Can you work these out from the model? Positions are in its coordinate system, mm. Round coordinates to 2 decimals unless told otherwise and drop trailing zeros. Loops run counter-clockwise (first coordinate to the right, second up) from the corner with the lowest first, then second, coordinate; pieces in that order, holes last.
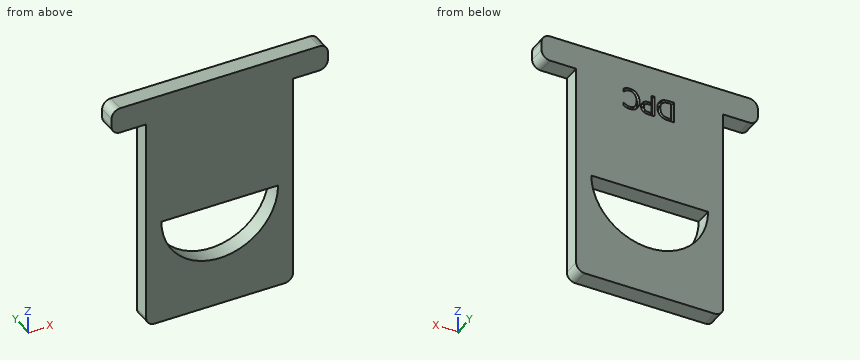
Autodesk Inventor part; units mm, degrees
ref_plane "YZ Plane" through (0, 0, 0) normal (1, 0, 0) x (0, 1, 0)
ref_plane "XZ Plane" through (0, 0, 0) normal (0, 1, 0) x (-1, 0, 0)
ref_plane "XY Plane" through (0, 0, 0) normal (0, 0, 1) x (1, 0, 0)
sketch "Sketch1" plane through (0, 0, 0) normal (0, 1, 0) x (-1, 0, 0)
  line L0 (-17, 25) -> (17, 25)
  line L1 (17, 25) -> (17, -25)
  line L2 (17, -25) -> (-17, -25)
  line L3 (-17, -25) -> (-17, 25)
  line L4 (-17, 25) -> (17, -25) construction
  line L5 (17, 25) -> (-17, -25) construction
  line L6 (9, -17) -> (9, 17)
  line L7 (9, 17) -> (-9, 17)
  line L8 (-9, 17) -> (-9, -17)
  line L9 (-9, -17) -> (9, -17)
  line L10 (-25, 31) -> (25, 31)
  line L11 (25, 31) -> (25, 25)
  line L12 (25, 25) -> (-25, 25)
  line L13 (-25, 25) -> (-25, 31)
  line L14 (-25, 31) -> (25, 25) construction
  line L15 (25, 31) -> (-25, 25) construction
  point P0 (0, 0)
  point P1 (0, 28)
  point P2 (0, 25)
  dimension "d0" = 34
  dimension "d1" = 50
  dimension "d2" = 8
  dimension "d3" = 50
  dimension "d4" = 6
extrude "Extrusion1" add sketch "Sketch1" along normal blind 4 contours L12 L13 L10 L11 L0 | L0 L1 L2 L3 | L9 L8 L7 L6
sketch "Sketch2" plane through (0, 4, 0) normal (0, 1, 0) x (1, 0, 0)
  line L0 (25, -25) -> (17, -25)
  line L1 (17, -25) -> (17, 25)
  line L2 (17, 25) -> (-17, 25)
  line L3 (-17, 25) -> (-17, -25)
  line L4 (-17, -25) -> (-25, -25)
  line L5 (-25, -25) -> (-25, -31)
  line L6 (-25, -31) -> (25, -31)
  line L7 (25, -31) -> (25, -25)
  line L8 (13.5, 17) -> (-13.5, 17)
  line L9 (-13.5, 17) -> (-13.5, -17)
  line L10 (-13.5, -17) -> (13.5, -17)
  line L11 (13.5, -17) -> (13.5, 17)
  line L12 (13.5, 17) -> (-13.5, -17) construction
  line L13 (-13.5, 17) -> (13.5, -17) construction
  circle A0 centre (0, 0.2783) radius 13.5
  line L14 (-13.5, 0.2783) -> (13.5, 0.2783)
  point P0 (-1.4697, 0.3)
  point P1 (1.4697, 0.3)
  point P2 (13.5, 0)
  point P3 (-13.5, 0)
  dimension "d7" = 27
  dimension "d8" = 34
extrude "Extrusion2" cut sketch "Sketch2" against normal through all contours L14 A0 picked at (2.5563, 3.9817)
sketch "Sketch3" plane through (0, 4, 0) normal (0, 1, 0) x (1, 0, 0)
  line L0 (-6.091, -19.1641) -> (19.1348, -19.1641) construction
  line L1 (19.1348, -19.1641) -> (19.1348, -24.3512) construction
  line L2 (19.1348, -24.3512) -> (-6.091, -24.3512) construction
  line L3 (-6.091, -24.3512) -> (-6.091, -19.1641) construction
  spline S0 degree 2 poles (-1.7599, -21.6886) (-1.7599, -22.3553) (-2.3003, -23.4282) (-2.7539, -23.728) knots 0 0 0 1 2 2 2
  spline S1 degree 2 poles (-2.7539, -23.728) (-3.1247, -23.9607) (-3.886, -24.1185) (-4.4777, -24.1185) knots 0 0 0 1 2 2 2
  line L4 (-4.4777, -24.1185) -> (-5.598, -24.1185)
  line L5 (-5.598, -24.1185) -> (-5.598, -19.2508)
  line L6 (-5.598, -19.2508) -> (-4.4895, -19.2508)
  spline S2 degree 2 poles (-4.4895, -19.2508) (-3.8032, -19.2508) (-3.0221, -19.456) (-2.746, -19.6374) knots 0 0 0 1 2 2 2
  spline S3 degree 2 poles (-2.746, -19.6374) (-2.2766, -19.949) (-1.7599, -20.9786) (-1.7599, -21.6886) knots 0 0 0 1 2 2 2
  spline S4 degree 2 poles (-2.4344, -21.6807) (-2.4344, -21.1206) (-2.8052, -20.3277) (-3.172, -20.1029) knots 0 0 0 1 2 2 2
  spline S5 degree 2 poles (-3.172, -20.1029) (-3.4324, -19.949) (-4.0201, -19.811) (-4.458, -19.811) knots 0 0 0 1 2 2 2
  line L7 (-4.458, -19.811) -> (-4.9511, -19.811)
  line L8 (-4.9511, -19.811) -> (-4.9511, -23.5584)
  line L9 (-4.9511, -23.5584) -> (-4.458, -23.5584)
  spline S6 degree 2 poles (-4.458, -23.5584) (-4.028, -23.5584) (-3.3772, -23.4203) (-3.1129, -23.2349) knots 0 0 0 1 2 2 2
  spline S7 degree 2 poles (-3.1129, -23.2349) (-2.7736, -23.0061) (-2.4344, -22.2488) (-2.4344, -21.6807) knots 0 0 0 1 2 2 2
  spline S8 degree 2 poles (2.0191, -20.7182) (2.0191, -21.0338) (1.7942, -21.6018) (1.5931, -21.7991) knots 0 0 0 1 2 2 2
  spline S9 degree 2 poles (1.5931, -21.7991) (1.3406, -22.0476) (0.6582, -22.304) (0.1375, -22.304) knots 0 0 0 1 2 2 2
  line L10 (0.1375, -22.304) -> (-0.4108, -22.304)
  line L11 (-0.4108, -22.304) -> (-0.4108, -24.1185)
  line L12 (-0.4108, -24.1185) -> (-1.0577, -24.1185)
  line L13 (-1.0577, -24.1185) -> (-1.0577, -19.2508)
  line L14 (-1.0577, -19.2508) -> (0.1651, -19.2508)
  spline S10 degree 2 poles (0.1651, -19.2508) (0.599, -19.2508) (1.2065, -19.3929) (1.4392, -19.5546) knots 0 0 0 1 2 2 2
  spline S11 degree 2 poles (1.4392, -19.5546) (1.7114, -19.74) (2.0191, -20.3119) (2.0191, -20.7182) knots 0 0 0 1 2 2 2
  spline S12 degree 2 poles (1.3446, -20.738) (1.3446, -20.4855) (1.171, -20.1147) (0.9935, -19.9964) knots 0 0 0 1 2 2 2
  spline S13 degree 2 poles (0.9935, -19.9964) (0.8396, -19.8938) (0.4294, -19.811) (0.1257, -19.811) knots 0 0 0 1 2 2 2
  line L15 (0.1257, -19.811) -> (-0.4108, -19.811)
  line L16 (-0.4108, -19.811) -> (-0.4108, -21.7517)
  line L17 (-0.4108, -21.7517) -> (0.031, -21.7517)
  spline S14 degree 2 poles (0.031, -21.7517) (0.4255, -21.7517) (0.9106, -21.6255) (1.0684, -21.4598) knots 0 0 0 1 2 2 2
  spline S15 degree 2 poles (1.0684, -21.4598) (1.2144, -21.3139) (1.3446, -20.9707) (1.3446, -20.738) knots 0 0 0 1 2 2 2
  spline S16 degree 2 poles (4.5357, -24.2053) (4.0624, -24.2053) (3.2616, -23.8858) (2.9697, -23.5663) knots 0 0 0 1 2 2 2
  spline S17 degree 2 poles (2.9697, -23.5663) (2.6778, -23.2507) (2.3583, -22.304) (2.3583, -21.6886) knots 0 0 0 1 2 2 2
  spline S18 degree 2 poles (2.3583, -21.6886) (2.3583, -21.0772) (2.6699, -20.1699) (2.9658, -19.8346) knots 0 0 0 1 2 2 2
  spline S19 degree 2 poles (2.9658, -19.8346) (3.2577, -19.5072) (4.0545, -19.1641) (4.5476, -19.1641) knots 0 0 0 1 2 2 2
  spline S20 degree 2 poles (4.5476, -19.1641) (4.7921, -19.1641) (5.2221, -19.2351) (5.4036, -19.2903) knots 0 0 0 1 2 2 2
  spline S21 degree 2 poles (5.4036, -19.2903) (5.5613, -19.3416) (5.8888, -19.4875) (6.0505, -19.5743) knots 0 0 0 1 2 2 2
  line L18 (6.0505, -19.5743) -> (6.0505, -20.3553)
  line L19 (6.0505, -20.3553) -> (5.9992, -20.3553)
  spline S22 degree 2 poles (5.9992, -20.3553) (5.9124, -20.2764) (5.6442, -20.0555) (5.4509, -19.949) knots 0 0 0 1 2 2 2
  spline S23 degree 2 poles (5.4509, -19.949) (5.2655, -19.8465) (4.8276, -19.7163) (4.5436, -19.7163) knots 0 0 0 1 2 2 2
  spline S24 degree 2 poles (4.5436, -19.7163) (4.232, -19.7163) (3.6758, -19.9727) (3.4668, -20.2173) knots 0 0 0 1 2 2 2
  spline S25 degree 2 poles (3.4668, -20.2173) (3.2616, -20.4658) (3.0328, -21.2192) (3.0328, -21.6886) knots 0 0 0 1 2 2 2
  spline S26 degree 2 poles (3.0328, -21.6886) (3.0328, -22.1896) (3.2735, -22.9114) (3.4825, -23.16) knots 0 0 0 1 2 2 2
  spline S27 degree 2 poles (3.4825, -23.16) (3.6877, -23.4006) (4.236, -23.6451) (4.5436, -23.6451) knots 0 0 0 1 2 2 2
  spline S28 degree 2 poles (4.5436, -23.6451) (4.8237, -23.6451) (5.301, -23.5071) (5.4864, -23.4045) knots 0 0 0 1 2 2 2
  spline S29 degree 2 poles (5.4864, -23.4045) (5.6639, -23.302) (5.9282, -23.089) (6.0031, -23.014) knots 0 0 0 1 2 2 2
  line L20 (6.0031, -23.014) -> (6.0505, -23.014)
  line L21 (6.0505, -23.014) -> (6.0505, -23.7872)
  spline S30 degree 2 poles (6.0505, -23.7872) (5.8888, -23.8621) (5.6047, -24.0002) (5.4036, -24.0633) knots 0 0 0 1 2 2 2
  spline S31 degree 2 poles (5.4036, -24.0633) (5.1906, -24.1343) (4.8276, -24.2053) (4.5357, -24.2053) knots 0 0 0 1 2 2 2
  point P0 (0, 0)
extrude "Extrusion3" cut sketch "Sketch3" against normal blind 1
fillet "Fillet1" radius 2 6 edges at (25, 2, 31) (25, 2, 25) (-25, 2, 31) (-25, 2, 25) (-17, 2, -25) (17, 2, -25)
properties part number "00_Slider_Mask_DPC"
(1) If we section it at B-B, the plane x = 11: List the corners of the cut face in (y, z) for me, then the cut area to 3 significant figures.
Worked answers:
outline: (0, -25) - (4, -25) - (4, -8.1) - (0, -8.1) - close; (0, -0.28) - (4, -0.28) - (4, 31) - (0, 31) - close
area: 193 mm2
(2) If we section it at C-C, the plane z = -8: List the corners of the cut face in (x, y) for me, then the cut area to 3 significant figures.
Worked answers:
outline: (-17, 0) - (-11.07, 0) - (-11.07, 4) - (-17, 4) - close; (11.07, 0) - (17, 0) - (17, 4) - (11.07, 4) - close
area: 47.4 mm2
(3) If we section it at D-D, the plane z = 16.5: List the corners of the cut face in (x, y) for me.
Worked answers:
outline: (-17, 0) - (17, 0) - (17, 4) - (-17, 4) - close
(4) If we section it at A-A, the plane y = 1.4: List the corners of the cut face in (x, z) for me.
Worked answers:
outline: (-25, 27) arc R2 ccw to (-23, 25) - (-17, 25) - (-17, -23) arc R2 ccw to (-15, -25) - (15, -25) arc R2 ccw to (17, -23) - (17, 25) - (23, 25) arc R2 ccw to (25, 27) - (25, 29) arc R2 ccw to (23, 31) - (-23, 31) arc R2 ccw to (-25, 29) - close; hole (-13.5, -0.28) arc R13.5 ccw to (13.5, -0.28) - close
(5) Will this pin go through, and if not, where does the flat tip stop? P1, Ø2, axis at y = 2.5, z = -2, coming from the +X side.
Worked answers:
P1: stops at x = 17
(6) If I drill on line 1 (X direction, y = 2.85, z = 4); line 2 (Z direction, x = -19, y = 3.55); line 3 (X direction, y = 1.75, z = -12), over which ranges is the centre line in solid material (lowest first)?
Worked answers:
line 1: x = -17 to 17
line 2: z = 25 to 31
line 3: x = -17 to -6.7, 6.7 to 17
